Read the model definition and answer for the solid it produces. Units are mm, in the model's axes. A direction names the side the tool comes from. Give positions to 0.01 mm unless a question says otherwise; leave off trailing zeros. Loops run counter-clockwise (first coordinate to the right, second up) from the corner with the lowest first, then second, coordinate; pieces in that order, holes last. Notation, with made-up numbers: (85.5, 87.5) - (141.5, 87.5) arc R27 ccw to (141.5, 118.5) - close; hole circle Ø7 at (-12.75, 14). An arc over 180 degrees is marked (long way). Write item = value, one per line. Start each with the question number.
from build123d import *

# Parameters (mm, degrees)
SKETCH1_W           = 19.05
SKETCH1_H           = 25.4
BOSS_EXTRUDE1_DEPTH = 5.08
SKETCH2_R           = 2.9972
CUT_EXTRUDE1_DEPTH  = 2.5146
SKETCH3_R           = 2.032
CUT_EXTRUDE2_DEPTH  = 3.5654
SKETCH4_R           = 1.2573
CUT_EXTRUDE4_DEPTH  = 6.08


with BuildPart() as part:
    # Sketch1 → Boss-Extrude1 (new body)
    with BuildSketch(Plane.XY):
        Rectangle(SKETCH1_W, SKETCH1_H)
    extrude(amount=BOSS_EXTRUDE1_DEPTH)

    # Sketch2 → Cut-Extrude1 (cut)
    with BuildSketch(Plane.XY.offset(5.08)):
        Circle(SKETCH2_R)
    extrude(amount=-CUT_EXTRUDE1_DEPTH, mode=Mode.SUBTRACT)

    # Sketch3 → Cut-Extrude2 (cut, through all)
    with BuildSketch(Plane.XY.offset(2.5654)):
        Circle(SKETCH3_R)
    extrude(amount=-CUT_EXTRUDE2_DEPTH, mode=Mode.SUBTRACT)

    # Sketch4 → Cut-Extrude4 (cut, through all)
    with BuildSketch(Plane.XY.offset(5.08)):
        with Locations((0, 5.5372)):
            Circle(SKETCH4_R)
        with Locations((5.5372, 0)):
            Circle(SKETCH4_R)
        with Locations((0, -5.5372)):
            Circle(SKETCH4_R)
        with Locations((-5.5372, 0)):
            Circle(SKETCH4_R)
    extrude(amount=-CUT_EXTRUDE4_DEPTH, mode=Mode.SUBTRACT)


solid = part.part
1. A cutting plane is placed at C-C on x = 6.25. Give the vertices of the cut face in (y, z).
2. A cutting plane is placed at A-A on x = 0. Give the vertices of the cut face in (y, z).
3. Consider line 1 along Y through (x, z) = (0, 3.45); line 2 along Y through (x, z) = (0, 2.2); line 3 along X through (y, z) = (6.25, 3.5) (3 decimals). Determine where each line is inside the solid, lowest interval first. Write a range as [from, to].
4. For a pull along X with two mould halves and no side action, classify faces 3 (the cylindrical face through (4.28, 0.06, 2.58)), 4 (the flat face through (9.525, 0, 3)), 5 (the flat face through (0, 12.7, 3)) as released by +X, released by -X, zero draft, split by the parting line, or undercut.
5. A tool of negligible diameter and unlimited length cuts with its end or side. For faces 1 (the flat face through (2, -1, 2.565)), 2 (the flat face through (2, 3, 5.08)), from which of +Z, -Z, +X, -X, +Y, -Y can it reach the whole face along a straight path? Write none if from no direction.
6. A cutting plane is placed at B-B on y = 0. Give the vertices of the cut face in (x, z) (1 decimal).
7. A cutting plane is placed at D-D on z = 0.8. Give the vertices of the cut face in (x, y) (1 decimal), and give its area (3 significant figures).
Reply:
q1.outline = (-12.7, 0) - (-1.04, 0) - (-1.04, 5.08) - (-12.7, 5.08) - close; (1.04, 0) - (12.7, 0) - (12.7, 5.08) - (1.04, 5.08) - close
q2.outline = (-12.7, 0) - (-6.79, 0) - (-6.79, 5.08) - (-12.7, 5.08) - close; (-4.28, 0) - (-2.03, 0) - (-2.03, 2.57) - (-3, 2.57) - (-3, 5.08) - (-4.28, 5.08) - close; (2.03, 0) - (4.28, 0) - (4.28, 5.08) - (3, 5.08) - (3, 2.57) - (2.03, 2.57) - close; (6.79, 0) - (12.7, 0) - (12.7, 5.08) - (6.79, 5.08) - close
q3.line_1 = [-12.7, -6.79], [-4.28, -3], [3, 4.28], [6.79, 12.7]
q3.line_2 = [-12.7, -6.79], [-4.28, -2.03], [2.03, 4.28], [6.79, 12.7]
q3.line_3 = [-9.525, -1.036], [1.036, 9.525]
q4.face_3 = undercut
q4.face_4 = released by +X
q4.face_5 = zero draft
q5.face_1 = +Z
q5.face_2 = +Z, +X, -X, +Y, -Y
q6.outline = (-9.5, 0) - (-6.8, 0) - (-6.8, 5.1) - (-9.5, 5.1) - close; (-4.3, 0) - (-2, 0) - (-2, 2.6) - (-3, 2.6) - (-3, 5.1) - (-4.3, 5.1) - close; (2, 0) - (4.3, 0) - (4.3, 5.1) - (3, 5.1) - (3, 2.6) - (2, 2.6) - close; (6.8, 0) - (9.5, 0) - (9.5, 5.1) - (6.8, 5.1) - close
q7.outline = (-9.5, -12.7) - (9.5, -12.7) - (9.5, 12.7) - (-9.5, 12.7) - close; hole circle Ø2.5 at (-5.5, 0); hole circle Ø4.1 at (0, 0); hole circle Ø2.5 at (0, -5.5); hole circle Ø2.5 at (0, 5.5); hole circle Ø2.5 at (5.5, 0)
q7.area = 451 mm^2
